Part model, mm, in its own coordinate system. Face numbers are marked on the shaded views. Round coordinates to 2 decimals unless told otherwise and drop trailing zeros. Write each loop counter-clockwise with the first axis right and the second up, starting at its lowest first coordinate (ties: lowest second). Pieces come first, ordered by that corner, then holes. Notation, with made-up numbers: (-4.5, -14.75) -> (19.5, -14.75) arc R11 ccw to (19.5, -6.75) -> close; hole circle Ø3 at (47.5, 64.5). An arc over 180 degrees is marked (long way). Return JSON: item names as keys, results as strings. Group by question number.
(1) Saw through at A-A (y = -201). List the corners of the cut face in (x, z).
(2) Saw through at C-C (x = -186.5). List the corners of the cut face in (y, z).
(3) Drill centre lines: L1, parallel to X at y = -407, z = 415; L2, parallel to Z at x = -7, y = -237; L3, parallel to Y at x = 180, z = 401. Where is each one in solid material? Low to high. Write a range as from..to.
(4) Saw through at B-B (z = 101.5). List the corners of the cut face in (x, y), plus the area to 3 significant figures.
(5) Drop a flat-ended pin along its axis: pin 1 Ø10 at (x, z) = (-83, 81.5) entering from -Y. Give the stop position or say it passes through.
(6) Mould opens along Y. For the marked faces 1, 2 and 3 say: +Y half, -Y half, draft (parallel to the pull), parting line (faces both ways), or undercut.
from build123d import *

# Parameters (mm, degrees)
F0_W     = 500
F0_H     = 1000
F1_DEPTH = 500
F2_T     = -12
F3_W     = 476
F3_H     = 38
F4_DEPTH = 20


with BuildPart() as f1:
    # F0 (on Top) → F1 (new body)
    with BuildSketch(Plane.XY):
        Rectangle(F0_W, F0_H)
    extrude(amount=F1_DEPTH)

    # F2
    f2_openings = [f1.faces().sort_by_distance(p)[0] for p in [
        (0, -500, 250),
    ]]
    offset(amount=F2_T, openings=f2_openings)

    # F3 (on face) → F4 (join)
    with BuildSketch(Plane.XZ.offset(500)):
        with Locations((0, 31)):
            Rectangle(F3_W, F3_H)
    extrude(amount=-F4_DEPTH)


solid = f1.part
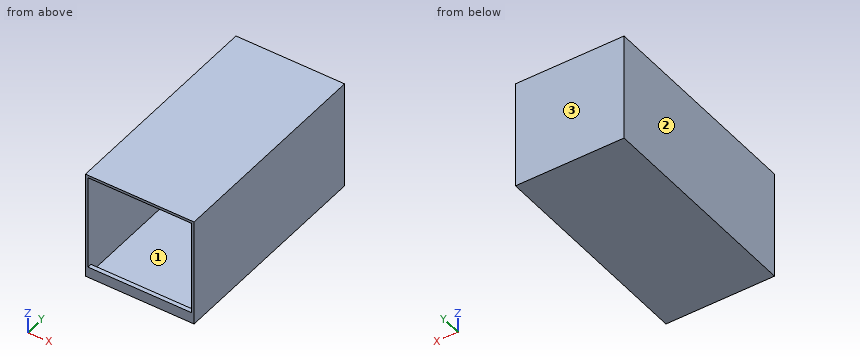
Computed values:
{
 "1": {"outline": "(-250, 0) -> (250, 0) -> (250, 500) -> (-250, 500) -> close; hole (-238, 12) -> (238, 12) -> (238, 488) -> (-238, 488) -> close"},
 "2": {"outline": "(-500, 0) -> (500, 0) -> (500, 500) -> (-500, 500) -> (-500, 488) -> (488, 488) -> (488, 12) -> (-480, 12) -> (-480, 50) -> (-500, 50) -> close"},
 "3": {"L1": "-250..-238, 238..250", "L2": "0..12, 488..500", "L3": "488..500"},
 "4": {"outline": "(-250, -500) -> (-238, -500) -> (-238, 488) -> (238, 488) -> (238, -500) -> (250, -500) -> (250, 500) -> (-250, 500) -> close", "area": "29,700 mm2"},
 "5": {"pin 1": "y = 488"},
 "6": {"face 1": "undercut", "face 2": "draft", "face 3": "+Y half"}
}
